For this review, take the finished solid that the model builds, in its own axes (mm). Face numbers are marked on the shaded views. A direction names the side the tool comes from. Round coordinates to 2 decimals unless told otherwise and drop trailing zeros. Order: outer loops, then holes, each group sorted by start corner. A loop starts at its lowest first (then second) coordinate and runs counter-clockwise, first axis right, second up. Notation, with made-up numbers: M 42.25,-29 L 54.25,-29 A31 cw 54.25,-1 Z; hole C 4,-13 d6. An arc over 180 degrees is marked long. Answer as a JSON object with one key per item and string values.
from build123d import *

# Parameters (mm, degrees)
F2_DEPTH = 5
F3_DEPTH = 5


with BuildPart() as f2:
    # F1 (on Top) → F2 (new body)
    with BuildSketch(Plane.XY):
        with BuildLine():
            ThreePointArc((7.560401775, -4.365), (8.4325324635, -2.2594902637), (8.73, 0))
            ThreePointArc((8.73, 0), (8.4325324635, 2.2594902637), (7.560401775, 4.365))
            ThreePointArc((7.560401775, 4.365), (-8.73, 0), (7.560401775, -4.365))
        make_face()
        with BuildLine():
            ThreePointArc((58.095, 0), (47.2143904114, 12.9064131387), (32.6539156005, 4.365))
            ThreePointArc((32.6539156005, 4.365), (31.905, 0), (32.6539156005, -4.365))
            ThreePointArc((32.6539156005, -4.365), (47.2143904114, -12.9064131387), (58.095, 0))
        make_face()
    extrude(amount=F2_DEPTH)

    # F1 (on Top) → F3 (join)
    with BuildSketch(Plane.XY):
        with BuildLine():
            ThreePointArc((58.095, 0), (47.2143904114, 12.9064131387), (32.6539156005, 4.365))
            ThreePointArc((32.6539156005, 4.365), (31.905, 0), (32.6539156005, -4.365))
            ThreePointArc((32.6539156005, -4.365), (47.2143904114, -12.9064131387), (58.095, 0))
        make_face()
        with BuildLine():
            ThreePointArc((7.560401775, 4.365), (8.4325324635, 2.2594902637), (8.73, 0))
            ThreePointArc((8.73, 0), (8.4325324635, -2.2594902637), (7.560401775, -4.365))
            Line((7.560401775, -4.365), (32.6539156005, -4.365))
            ThreePointArc((32.6539156005, -4.365), (31.905, 0), (32.6539156005, 4.365))
            Line((32.6539156005, 4.365), (7.560401775, 4.365))
        make_face()
        with BuildLine():
            ThreePointArc((7.560401775, -4.365), (8.4325324635, -2.2594902637), (8.73, 0))
            ThreePointArc((8.73, 0), (8.4325324635, 2.2594902637), (7.560401775, 4.365))
            ThreePointArc((7.560401775, 4.365), (-8.73, 0), (7.560401775, -4.365))
        make_face()
    extrude(amount=-F3_DEPTH)


with BuildPart() as f2_1:
    # F4: moved
    add(f2.part.moved(Location((0, 0, -5))))


solid = f2_1.part
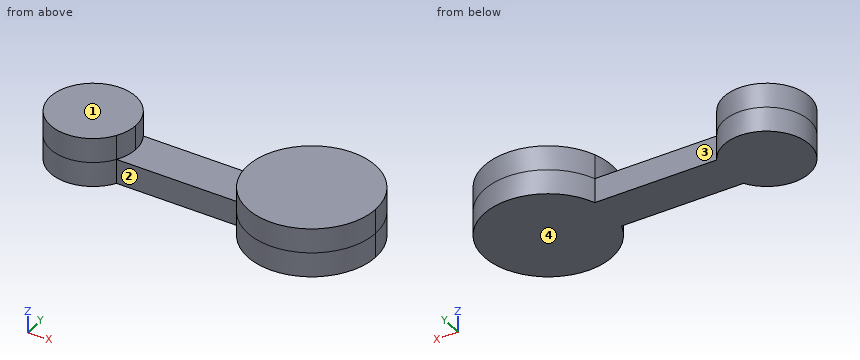
1) Add section B-B on z = -7.5. State the section outline as (x, y) points (3 decimals), and give its area (3 significant figures).
Geometry check:
{"outline": "M 7.56,-4.365 L 32.654,-4.365 A13.095 ccw long 32.654,4.365 L 7.56,4.365 A8.73 ccw long Z", "area": "986 mm²"}
2) Add section C-C on x = 23. State the section outline as (y, z) points (3 decimals).
Geometry check:
{"outline": "M -4.365,-10 L 4.365,-10 L 4.365,-5 L -4.365,-5 Z"}
3) Machinability: for the marked faces 1 and 2, which of the approach directions +Z, -Z, +X, -X, +Y, -Y give a long, thin tool a straight path to every point of the face, cutting with its end or side? Answer none if there is none.
Geometry check:
{"face 1": "+Z, +X, -X, +Y, -Y", "face 2": "+Z, -Z, -Y"}
4) Insertion check: P1, Ø4.5, axis at x = 20, y = -1, coming from the +Z side; P2, Ø1.5, axis at x = 36, z = -8, coming from the +Y side; P3, Ø1.5, axis at x = 19, z = -7, coming from the -Y side (3 decimals). Each pin has a flat end and moves straight along its axis. Give the tip position at first contact, or say it passes through.
Geometry check:
{"P1": "stops at z = -5", "P2": "stops at y = 10.17", "P3": "stops at y = -4.365"}
5) Mouldability with a two-part tool opening along X and no side actions: class the marked faces 3 and 4 as +X half, -X half, draft (parallel to the pull), parting line (faces both ways), or undercut.
Geometry check:
{"face 3": "undercut", "face 4": "draft"}
6) For L1, parallel to Y at x = 17, z = -8.75 (3 decimals); L2, parallel to Z at x = 31, y = -1.5; L3, parallel to X at y = 6.25, z = -7.5, list the stretches that pass through material, from the lowest coordinate up.
Geometry check:
{"L1": "y = -4.365 to 4.365", "L2": "z = -10 to -5", "L3": "x = -6.1 to 6.1, 33.49 to 56.51"}
7) Add section A-A on x = 0. State the section outline as (y, z) points.
Geometry check:
{"outline": "M -8.73,-10 L 8.73,-10 L 8.73,0 L -8.73,0 Z"}
